Verification items for the finished model (mm, model axes). A direction names the side the tool comes from. Round coordinates to 2 decimals unless told otherwise and drop trailing zeros. Order: outer loops, then holes, each group sorted by start corner. A loop starts at its lowest first (then second) coordinate and runs counter-clockwise, first axis right, second up. Notation, with made-up numbers: (84.5, 33) -> (95.5, 33) arc R20 cw to (95.5, 46) -> close; hole circle Ø3 at (8.5, 37). An arc over 180 degrees is marked (long way). Answer in a Markdown table with one row per item. Add a question column.
```python
from build123d import *

# Parameters (mm, degrees)
SKETCH1_W               = 203.2
SKETCH1_H               = 152.4
BOSS_EXTRUDE2_DEPTH     = 5.334
SKETCH2_R               = 18
SKETCH2_R_2             = 1.575
CUT_EXTRUDE1_DEPTH      = 184.239656068
SKETCH3_W               = 24.13
SKETCH3_H               = 5.08
BOSS_EXTRUDE3_DEPTH     = 5.334
SKETCH4_W               = 5.842
SKETCH4_H               = 12.954
CUT_EXTRUDE2_DEPTH      = 184.239656068
MIRROR3_COPY_1_SKETCH_W = 24.13
MIRROR3_COPY_1_SKETCH_H = 5.08
MIRROR3_COPY_1_DEPTH    = 5.334


with BuildPart() as part:
    # Sketch1 → Boss-Extrude2 (new body)
    with BuildSketch(Plane(origin=(0, 0, 0), x_dir=(0, 0, -1), z_dir=(1, 0, 0))):
        with Locations((0, 76.2)):
            Rectangle(SKETCH1_W, SKETCH1_H)
    extrude(amount=BOSS_EXTRUDE2_DEPTH)

    # Sketch2 → Cut-Extrude1 (cut, through all)
    with BuildSketch(Plane.ZY):
        with Locations((0, 76.2)):
            Circle(SKETCH2_R)
        with Locations((-15.5, 91.7)):
            Circle(SKETCH2_R_2)
        with Locations((15.5, 91.7)):
            Circle(SKETCH2_R_2)
        with Locations((15.5, 60.7)):
            Circle(SKETCH2_R_2)
        with Locations((-15.5, 60.7)):
            Circle(SKETCH2_R_2)
    extrude(amount=-CUT_EXTRUDE1_DEPTH, mode=Mode.SUBTRACT)

    # Sketch3 → Boss-Extrude3 (add, through all)
    with BuildSketch(Plane(origin=(5.334, 0, 0), x_dir=(0, 0, -1), z_dir=(1, 0, 0))):
        with Locations((69.85, -2.54)):
            Rectangle(SKETCH3_W, SKETCH3_H)
    boss_extrude3 = extrude(amount=-BOSS_EXTRUDE3_DEPTH)

    # Mirror1: Boss-Extrude3 across plane
    add(boss_extrude3.mirror(Plane.XY))

    # Sketch4 → Cut-Extrude2 (cut, through all)
    with BuildSketch(Plane(origin=(5.334, 0, 0), x_dir=(0, 0, -1), z_dir=(1, 0, 0))):
        with Locations((73.025, 25.3365)):
            Rectangle(SKETCH4_W, SKETCH4_H)
        with Locations((73.025, 53.9115)):
            Rectangle(SKETCH4_W, SKETCH4_H)
    cut_extrude2 = extrude(amount=-CUT_EXTRUDE2_DEPTH, mode=Mode.SUBTRACT)

    # Mirror2: Cut-Extrude2 across plane
    add(cut_extrude2.mirror(Plane.XY), mode=Mode.SUBTRACT)

    # Mirror3: Boss-Extrude3 across plane
    add(boss_extrude3.mirror(Plane(origin=(0, 76.2, 0), x_dir=(0, 0, 1), z_dir=(0, -1, 0))))

    # Mirror3 copy 1 sketch → Mirror3 copy 1 (add, through all)
    with BuildSketch(Plane(origin=(5.334, 152.4, 0), x_dir=(0, 0, 1), z_dir=(1, 0, 0))):
        with Locations((69.85, -2.54)):
            Rectangle(MIRROR3_COPY_1_SKETCH_W, MIRROR3_COPY_1_SKETCH_H)
    extrude(amount=-MIRROR3_COPY_1_DEPTH)


solid = part.part
```
1) Cross-section at C-C, the plane x = 3.3. Give the number of separate pieces and of enclosed holes in the cut face, and give its area (3 significant figures).
2) Cross-section at B-B, the plane z = 0. Record the boundary of the cut face in (x, y).
3) Depth check by flat-ended pin: P1, Ø4, axis at y = 34.5, z = -4, coming from the -X side; P2, Ø1.5, axis at x = 4, z = 47.5, coming from the -Y side; P3, Ø1.6, axis at x = 3.5, z = 91.5, coming from the +Y side. Enter the tip coordinate at first touch or a pass-through.
4) Cross-section at A-A, the plane y = 76.2. Record the boundary of the cut face in (x, z).
5) Cross-section at D-D, the plane z = 52.5. Record the boundary of the cut face in (x, y).
6) Tool access check on faces 1 (the face through (3, 0, -92)), 2 (the face through (3, 152.4, 92)), 3 (the face through (3, 31.814, -73)), 4 (the face through (3, 0, 92)), 5 (the face through (3, 155, -81.915)). Record the directions out of +Z, -Z, +X, -X, +Y, -Y that give a thin tool (end or side, any length) a straight path to the whole face; none if there is none.
7) Draft check along Z on faces 6 (the face through (3, 54, 75.946)), 7 (the face through (3, 75, 101.6)), 8 (the face through (3, 157.48, -70)). Enter one of: +Z half, -Z half, draft (parallel to the pull), parting line (faces both ways), or undercut.
8) Thickness scan on L1, parallel to Z at x = 1.85, y = 53; L2, parallel to Y at x = 2.25, z = -15.5 (1 decimal); L3, parallel to Z at x = 2.15, y = 91.7 (1 decimal). Record the ranges inside material, lowest first. Write a range as [from, to].
Results below:
| question | item | result |
|---|---|---|
| 1 | separate pieces | 1 |
| 1 | enclosed holes | 9 |
| 1 | area | 30,100 mm² |
| 2 | outline | (0, 0) -> (5.33, 0) -> (5.33, 58.2) -> (0, 58.2) -> close; (0, 94.2) -> (5.33, 94.2) -> (5.33, 152.4) -> (0, 152.4) -> close |
| 3 | P1 | x = 0 |
| 3 | P2 | y = 0 |
| 3 | P3 | y = 152.4 |
| 4 | outline | (0, -101.6) -> (5.33, -101.6) -> (5.33, -18) -> (0, -18) -> close; (0, 18) -> (5.33, 18) -> (5.33, 101.6) -> (0, 101.6) -> close |
| 5 | outline | (0, 0) -> (5.33, 0) -> (5.33, 152.4) -> (0, 152.4) -> close |
| 6 | face 1 | -Z, +X, -X, -Y |
| 6 | face 2 | +Z, +X, -X, +Y |
| 6 | face 3 | +X, -X |
| 6 | face 4 | +Z, +X, -X, -Y |
| 6 | face 5 | -Z, +X, -X, +Y |
| 7 | face 6 | undercut |
| 7 | face 7 | +Z half |
| 7 | face 8 | draft |
| 8 | L1 | [-101.6, -75.95], [-70.1, 70.1], [75.95, 101.6] |
| 8 | L2 | [0, 59.1], [62.3, 67], [85.4, 90.1], [93.3, 152.4] |
| 8 | L3 | [-101.6, -17.1], [-13.9, -9.2], [9.2, 13.9], [17.1, 101.6] |
